from build123d import *

# Parameters (mm, degrees)
CROQUIS1_R              = 2.950001172
CROQUIS1_W              = 9
CROQUIS1_H              = 9
SALIENTE_EXTRUIR1_DEPTH = 3
SALIENTE_EXTRUIR6_DEPTH = 5


with BuildPart() as part:
    # Croquis1 → Saliente-Extruir1 (new body)
    with BuildSketch(Plane.XY.offset(-0.156260387)):
        Polygon((51.261125499, 62.988673094), (44.261125499, 69.988673094), (-35.738874501, 69.988673094), (-42.738874501, 62.988673094), (-45.738874501, 62.988673094), (-45.738874501, -27.011326906), (54.261125499, -27.011326906), (54.261125499, 62.988673094), align=None)
        with Locations((7.161124531, 48.770443145)):
            Circle(CROQUIS1_R, mode=Mode.SUBTRACT)
        with Locations((28.761125092, 35.170443896)):
            Circle(CROQUIS1_R, mode=Mode.SUBTRACT)
        with Locations((28.761125092, 14.5704435)):
            Circle(CROQUIS1_R, mode=Mode.SUBTRACT)
        with Locations((6.661127243, -6.529559074)):
            Circle(CROQUIS1_R, mode=Mode.SUBTRACT)
        with Locations((-15.198872503, 14.470443669)):
            Circle(CROQUIS1_R, mode=Mode.SUBTRACT)
        with Locations((-15.738875683, 34.170445595)):
            Circle(CROQUIS1_R, mode=Mode.SUBTRACT)
        with Locations((7.748576734, 31.892113927)):
            Rectangle(CROQUIS1_W, CROQUIS1_H, mode=Mode.SUBTRACT)
    extrude(amount=SALIENTE_EXTRUIR1_DEPTH)

    # Croquis9 → Saliente-Extruir6 (add)
    with BuildSketch(Plane(origin=(0, 0, -0.156260387), x_dir=(-1, 0, 0), z_dir=(0, 0, -1))):
        Polygon((-51.261125499, 62.988673094), (-48.261125499, 62.988673094), (-48.261125499, -21.011326906), (39.738874501, -21.011326906), (39.738874501, 62.988673094), (42.738874501, 62.988673094), (42.738874501, -24.011326906), (-51.261125499, -24.011326906), align=None)
    extrude(amount=SALIENTE_EXTRUIR6_DEPTH)


solid = part.part
Model file for the job. Use its own axes, mm. A direction names the side the tool comes from. Coordinates: 2 decimals unless noted, no trailing zeros. Order: outer loops, then holes, each group sorted by start corner. A loop starts at its lowest first (then second) coordinate and runs counter-clockwise, first axis right, second up. Notation, with made-up numbers: (-4.5, 52) -> (26.5, 52) arc R19 ccw to (26.5, 76) -> close; hole circle Ø11 at (-9, 11.25). An arc over 180 degrees is marked (long way). Return JSON: item names as keys, results as strings. Group by question number.
Item 1: Saw through at B-B on y = -8. Write the cut outline in (x, z).
Item 2: Tool access for faces 4 (the flat face through (-42.739, 20, -3)), 5 (the flat face through (53, 62.989, 1)), 6 (the flat face through (-44, 62.989, 1)): list every direction of +Z, -Z, +X, -X, +Y, -Y with a clear straight run to the whole face (end or side of a thin tool).
Item 3: Pull direction X, two halves, no side cores. Call faces 1 (the flat face through (4, -24.011, -3)), 2 (the cylindrical face through (25.814, 14.7, 1.323)), 3 (the flat face through (51.261, 19, -3)): pulls with the +X half, pulls with the -X half, needs draft (parallel to the pull), parting line crosses it, or undercut.
Item 4: Saw through at A-A on x = -32. Write the cut outline in (y, z), then the cut area to 3 significant figures.
Item 5: Wall check: line 1 along X through (y, z) = (17, -3.75); line 2 along Y through (x, z) = (27, 0); line 3 along Z through (x, y) = (36.5, -7.5). Give the ranges that are in metal, low to high. Write a range as [from, to].
Item 6: Saw through at D-D on y = 61. Write the cut outline in (x, z), then the cut area to 3 significant figures.
Item 7: Flat gauge pins, fed straight in: P1, Ø1, axis at y = 24.5, z = -2.5, coming from the +X side; P2, Ø2.5, axis at y = 21.5, z = -3, coming from the -X side; P3, Ø2, axis at x = 8, z = -1.5, coming from the -Y side. Where does each tip first touch, or does it go through?
Item 8: Saw through at C-C on z = 1. Write the cut outline in (x, y).
Values found:
{
 "1": {"outline": "(-45.74, -0.16) -> (-42.74, -0.16) -> (-42.74, -5.16) -> (-39.74, -5.16) -> (-39.74, -0.16) -> (4.1, -0.16) -> (4.1, 2.84) -> (-45.74, 2.84) -> close; (9.22, -0.16) -> (48.26, -0.16) -> (48.26, -5.16) -> (51.26, -5.16) -> (51.26, -0.16) -> (54.26, -0.16) -> (54.26, 2.84) -> (9.22, 2.84) -> close"},
 "2": {"face 4": "-Z, -X, +Y, -Y", "face 5": "+Z, -Z, +X, +Y", "face 6": "+Z, -Z, -X, +Y"},
 "3": {"face 1": "needs draft", "face 2": "undercut", "face 3": "pulls with the +X half"},
 "4": {"outline": "(-27.01, -0.16) -> (-24.01, -0.16) -> (-24.01, -5.16) -> (-21.01, -5.16) -> (-21.01, -0.16) -> (69.99, -0.16) -> (69.99, 2.84) -> (-27.01, 2.84) -> close", "area": "306 mm2"},
 "5": {"line 1": "x = [-42.74, -39.74], [48.26, 51.26]", "line 2": "y = [-27.01, 12.2], [16.94, 32.8], [37.54, 69.99]", "line 3": "z = [-0.16, 2.84]"},
 "6": {"outline": "(-45.74, -0.16) -> (-42.74, -0.16) -> (-42.74, -5.16) -> (-39.74, -5.16) -> (-39.74, -0.16) -> (48.26, -0.16) -> (48.26, -5.16) -> (51.26, -5.16) -> (51.26, -0.16) -> (54.26, -0.16) -> (54.26, 2.84) -> (-45.74, 2.84) -> close", "area": "330 mm2"},
 "7": {"P1": "stops at x = 51.26", "P2": "stops at x = -42.74", "P3": "stops at y = -24.01"},
 "8": {"outline": "(-45.74, -27.01) -> (54.26, -27.01) -> (54.26, 62.99) -> (51.26, 62.99) -> (44.26, 69.99) -> (-35.74, 69.99) -> (-42.74, 62.99) -> (-45.74, 62.99) -> close; hole circle Ø5.9 at (-15.74, 34.17); hole circle Ø5.9 at (-15.2, 14.47); hole (3.25, 27.39) -> (12.25, 27.39) -> (12.25, 36.39) -> (3.25, 36.39) -> close; hole circle Ø5.9 at (6.66, -6.53); hole circle Ø5.9 at (7.16, 48.77); hole circle Ø5.9 at (28.76, 14.57); hole circle Ø5.9 at (28.76, 35.17)"}
}
